Source: CAD feature listing. Evaluate the final solid. Frame: model axes, mm. A direction names the side the tool comes from. Give positions to 0.01 mm unless a question says otherwise; leave off trailing zeros.
from build123d import *
from build123d.topology import SkipClean

# Parameters (mm, degrees)
CROQUIS1_R               = 1.65
SALIENTE_EXTRUIR1_DEPTH  = 1
CROQUIS3_W               = 30
CROQUIS3_H               = 2
SALIENTE_EXTRUIR2_DEPTH  = 13
CROQUIS4_R               = 1.55
CORTAR_EXTRUIR1_DEPTH    = 64.41135545
CROQUIS8_W               = 11
CROQUIS8_H               = 23.108
SALIENTE_EXTRUIR4_DEPTH  = 1
SALIENTE_EXTRUIR5_DEPTH  = 16
CORTAR_EXTRUIR2_DEPTH    = 46.124826869
SALIENTE_EXTRUIR6_DEPTH  = 5
CROQUIS12_R              = 1
CORTAR_EXTRUIR3_DEPTH    = 5
CROQUIS13_W              = 2
CROQUIS13_H              = 56
SALIENTE_EXTRUIR7_DEPTH  = 1.5
SALIENTE_EXTRUIR8_DEPTH  = 2
CROQUIS15_W              = 2
CROQUIS15_H              = 1.5
SALIENTE_EXTRUIR9_DEPTH  = 5
NERVIO4_REACH            = 54.69
CROQUIS16_WALL_W         = 115.107854894
CROQUIS16_WALL_H         = 1
NERVIO5_REACH            = 56.037
CROQUIS17_WALL_W         = 121.609320684
CROQUIS17_WALL_H         = 2
SALIENTE_EXTRUIR10_DEPTH = 1
MATRIZL1_COUNT           = 2
MATRIZL1_PITCH           = 6
NERVIO9_REACH            = 63.857
CROQUIS19_WALL_W         = 137.248650414
CROQUIS19_WALL_H         = 2
NERVIO10_REACH           = 63.857
CROQUIS20_WALL_W         = 136.67923452
CROQUIS20_WALL_H         = 2
REDONDEO1_R              = 1.5
CROQUIS21_R              = 5
CORTAR_EXTRUIR4_DEPTH    = 2


with BuildPart() as part:
    # Croquis1 → Saliente-Extruir1 (new body)
    with BuildSketch(Plane(origin=(0, 0, 0), x_dir=(0, 0, -1), z_dir=(1, 0, 0))):
        Polygon((-15, 18), (-15, -18), (15, -18), (15, 18), (15, 42), (-15, 42), align=None)
        with Locations((0, 12.5)):
            Circle(CROQUIS1_R, mode=Mode.SUBTRACT)
        with Locations((0, -12.5)):
            Circle(CROQUIS1_R, mode=Mode.SUBTRACT)
    extrude(amount=SALIENTE_EXTRUIR1_DEPTH)

    # Croquis3 → Saliente-Extruir2 (add)
    with BuildSketch(Plane(origin=(1, 0, 0), x_dir=(0, 0, -1), z_dir=(1, 0, 0))):
        with Locations((0, 41)):
            Rectangle(CROQUIS3_W, CROQUIS3_H)
        with Locations((0, -17)):
            Rectangle(CROQUIS3_W, CROQUIS3_H)
    extrude(amount=SALIENTE_EXTRUIR2_DEPTH)

    # Croquis4 → Cortar-Extruir1 (cut, through all)
    with BuildSketch(Plane(origin=(0, 42, 0), x_dir=(1, 0, 0), z_dir=(0, 1, 0))):
        with Locations(Location((10, 7.5, 0), (0, 0, 270))):
            Circle(CROQUIS4_R)
        with Locations(Location((10, -7.5, 0), (0, 0, 270))):
            Circle(CROQUIS4_R)
        with BuildLine():
            Line((14, 5.656854249), (14, -5.656854249))
            ThreePointArc((14, -5.656854249), (10, 0), (14, 5.656854249))
        make_face()
    extrude(amount=-CORTAR_EXTRUIR1_DEPTH, mode=Mode.SUBTRACT)

    # Croquis8 → Saliente-Extruir4 (add)
    with BuildSketch(Plane(origin=(0, 0, 0), x_dir=(0, 0, -1), z_dir=(1, 0, 0))):
        with Locations((-20.5, 0.946)):
            Rectangle(CROQUIS8_W, CROQUIS8_H)
    extrude(amount=SALIENTE_EXTRUIR4_DEPTH)

    # Croquis9 → Saliente-Extruir5 (add)
    with BuildSketch(Plane(origin=(0, 0, 0), x_dir=(0, 0, -1), z_dir=(1, 0, 0))):
        Polygon((-26, -10.608), (-26, 12.5), (-15, 12.5), (-15, 14), (-27.5, 14), (-27.5, -12.108), (-15, -12.108), (-15, -10.608), align=None)
    extrude(amount=SALIENTE_EXTRUIR5_DEPTH)

    # Croquis10 → Cortar-Extruir2 (cut, through all)
    with BuildSketch(Plane(origin=(0, 14, 0), x_dir=(1, 0, 0), z_dir=(0, 1, 0))):
        with BuildLine():
            ThreePointArc((4.5, -21.25), (3.369306394, -19.158349934), (1, -18.958712153))
            Line((1, -18.958712153), (1, -23.541287847))
            ThreePointArc((1, -23.541287847), (3.369306394, -23.341650066), (4.5, -21.25))
        make_face()
    extrude(amount=-CORTAR_EXTRUIR2_DEPTH, mode=Mode.SUBTRACT)

    # Croquis11 → Saliente-Extruir6 (add)
    with BuildSketch(Plane(origin=(16, 0, 0), x_dir=(0, 0, -1), z_dir=(1, 0, 0))):
        with BuildLine():
            Line((-21.435245422, -12.108), (-22.974809892, -12.108))
            ThreePointArc((-22.974809892, -12.108), (-20.5, -14.254), (-18.025190108, -12.108))
            Line((-18.025190108, -12.108), (-19.564754578, -12.108))
            ThreePointArc((-19.564754578, -12.108), (-20.5, -12.754), (-21.435245422, -12.108))
        make_face()
        with BuildLine():
            ThreePointArc((-18.025190108, 14), (-20.5, 16.146), (-22.974809892, 14))
            Line((-22.974809892, 14), (-21.435245422, 14))
            ThreePointArc((-21.435245422, 14), (-20.5, 14.646), (-19.564754578, 14))
            Line((-19.564754578, 14), (-18.025190108, 14))
        make_face()
    extrude(amount=-SALIENTE_EXTRUIR6_DEPTH)

    # Croquis12 → Cortar-Extruir3 (cut)
    with BuildSketch(Plane(origin=(16, 0, 0), x_dir=(0, 0, -1), z_dir=(1, 0, 0))):
        with Locations((-20.5, -11.754)):
            Circle(CROQUIS12_R)
        with Locations((-20.5, 13.646)):
            Circle(CROQUIS12_R)
    extrude(amount=-CORTAR_EXTRUIR3_DEPTH, mode=Mode.SUBTRACT)

    # Croquis13 → Saliente-Extruir7 (add)
    with BuildSketch(Plane(origin=(1, 0, 0), x_dir=(0, 0, -1), z_dir=(1, 0, 0))):
        with Locations((-14, 12)):
            Rectangle(CROQUIS13_W, CROQUIS13_H)
        with Locations((14, 12)):
            Rectangle(CROQUIS13_W, CROQUIS13_H)
    extrude(amount=SALIENTE_EXTRUIR7_DEPTH)

    # Croquis14 → Saliente-Extruir8 (add)
    with BuildSketch(Plane(origin=(0, 0, 15), x_dir=(-1, 0, 0), z_dir=(0, 0, -1))):
        Polygon((-12.5, 12.5), (-2.5, 19), (-2.5, 12.5), align=None)
    extrude(amount=SALIENTE_EXTRUIR8_DEPTH)

    # Croquis15 → Saliente-Extruir9 (add)
    with BuildSketch(Plane(origin=(14, 0, 0), x_dir=(0, 0, -1), z_dir=(1, 0, 0))):
        with Locations((-14, 13.25)):
            Rectangle(CROQUIS15_W, CROQUIS15_H)
    extrude(amount=-SALIENTE_EXTRUIR9_DEPTH)

    # Croquis16 wall → Nervio4 (add, up to next)
    with BuildSketch(Plane(origin=(0, -15.054, 17.5), x_dir=(0, -0.76246270462, -0.647032166174), z_dir=(0, -0.647032166174, 0.76246270462)), mode=Mode.PRIVATE) as nervio4_sk1:
        with Locations((0, 0.5)):
            Rectangle(CROQUIS16_WALL_W, CROQUIS16_WALL_H)
    nervio4_tool1 = extrude(nervio4_sk1.sketch, amount=-NERVIO4_REACH, mode=Mode.PRIVATE) - part.part
    add(nervio4_tool1.solids().sort_by_distance((0, -15.054, 17.5))[0])

    # Croquis17 wall → Nervio5 (add, up to next)
    with BuildSketch(Plane(origin=(5.375, 35, 15), x_dir=(-0.498471124258, -0.866906303058, 0), z_dir=(0.866906303058, -0.498471124258, 0)), mode=Mode.PRIVATE) as nervio5_sk1:
        with Locations((0, 1)):
            Rectangle(CROQUIS17_WALL_W, CROQUIS17_WALL_H)
    nervio5_tool1 = extrude(nervio5_sk1.sketch, amount=-NERVIO5_REACH, mode=Mode.PRIVATE) - part.part
    add(nervio5_tool1.solids().sort_by_distance((5.375, 35, 15))[0])

    # Croquis18 → Saliente-Extruir10 (add)
    with SkipClean():  # the faces are left unmerged after this step: merging them gives an invalid solid
        with BuildSketch(Plane(origin=(14, 0, 0), x_dir=(0, 0, -1), z_dir=(1, 0, 0))):
            with BuildLine():
                Line((-15, -18), (-19.744471073, -12.409115288))
                ThreePointArc((-19.744471073, -12.409115288), (-19.641310837, -12.266496752), (-19.564754578, -12.108))
                Line((-19.564754578, -12.108), (-15, -12.108))
                Line((-15, -12.108), (-15, -18))
            make_face()
        saliente_extruir10 = extrude(amount=-SALIENTE_EXTRUIR10_DEPTH)

    # MatrizL1: Saliente-Extruir10 ×2
    with SkipClean():  # the faces are left unmerged after this step: merging them gives an invalid solid
        with Locations(*[(-i * MATRIZL1_PITCH, 0, 0) for i in range(1, MATRIZL1_COUNT)]):
            add(saliente_extruir10)

    # Croquis19 wall → Nervio9 (add, up to next)
    with BuildSketch(Plane(origin=(5.375, 35, -15), x_dir=(-0.498471124258, -0.866906303058, 0), z_dir=(-0.866906303058, 0.498471124258, 0)), mode=Mode.PRIVATE) as nervio9_sk1:
        with Locations((0, 1)):
            Rectangle(CROQUIS19_WALL_W, CROQUIS19_WALL_H)
    nervio9_tool1 = extrude(nervio9_sk1.sketch, amount=NERVIO9_REACH, mode=Mode.PRIVATE) - part.part
    add(nervio9_tool1.solids().sort_by_distance((5.375, 35, -15))[0])

    # Croquis20 wall → Nervio10 (add, up to next)
    with BuildSketch(Plane(origin=(4.75, -11, -15), x_dir=(-0.410364677329, 0.911921505175, 0), z_dir=(0.911921505175, 0.410364677329, 0)), mode=Mode.PRIVATE) as nervio10_sk1:
        with Locations((0, 1)):
            Rectangle(CROQUIS20_WALL_W, CROQUIS20_WALL_H)
    nervio10_tool1 = extrude(nervio10_sk1.sketch, amount=-NERVIO10_REACH, mode=Mode.PRIVATE) - part.part
    add(nervio10_tool1.solids().sort_by_distance((4.75, -11, -15))[0])

    # Redondeo1
    redondeo1_edges = [part.edges().sort_by_distance(p)[0] for p in [
        (5.096153846, 14, 15),
        (1, 40, 0),
        (1, 12, 13),
        (1, -16, 0),
        (1, 12, -13),
    ]]
    fillet(redondeo1_edges, radius=REDONDEO1_R - 0.0001)  # a hair under: the kernel refuses the full size

    # Croquis21 → Cortar-Extruir4 (cut)
    with BuildSketch(Plane.XY.offset(27.5)):
        with Locations((8, 0)):
            Circle(CROQUIS21_R)
    extrude(amount=-CORTAR_EXTRUIR4_DEPTH, mode=Mode.SUBTRACT)


solid = part.part
1) Contact query for flat-ended pins moving along their axis: P1, Ø5.5, axis at y = -12.5, z = 0, coming from the +X side; P2, Ø4, axis at x = 12.5, z = 16, coming from the -Y side; P3, Ø1.1, axis at y = -11.5, z = 20.5, coming from the +X side; P4, Ø1.1, axis at y = -13.5, z = 20.5, coming from the -X side. Output: stop coordinate, or through.
Checks:
P1: stops at x = 1.2
P2: stops at y = -18
P3: stops at x = 11
P4: stops at x = 11
2) Reachability of faces 1 (the flat face through (7.51, -15.24, 17.34)), 2 (the flat face through (11, -13, 21)), 3 (the flat face through (1, -1, 19)), 4 (the flat face through (3, 33, -13)) from +Z, -Z, +X, -X, +Y, -Y: full face, straight path, thin tool, end or side. Return the list, or none.
Checks:
face 1: +Z, -X, -Y
face 2: +Z, -Z, -Y
face 3: none
face 4: +X
3) Ray query, probe 1 along Y at (x, z) = (0.35, 0); probe 2 along X at (y, z) = (40.65, -7.5); probe 3 along Y at (x, z) = (8, 26.7). Return the intervals inside material, ascending.
Checks:
probe 1: y = -18 to -14.15, -10.85 to 10.85, 14.15 to 42
probe 2: x = 0 to 8.45, 11.55 to 14
probe 3: y = -12.11 to -5, 5 to 14
4) Pull-direction query (Y, two-part tool) for faces 5 (the flat face through (16, 2.1, 26.4)), 6 (the flat face through (7, 42, 0)), 7 (the flat face through (5.415, 35.07, -13.986)); classes: released by +Y, released by -Y, zero draft, split by the parting line, or undercut.
Checks:
face 5: zero draft
face 6: released by +Y
face 7: undercut
